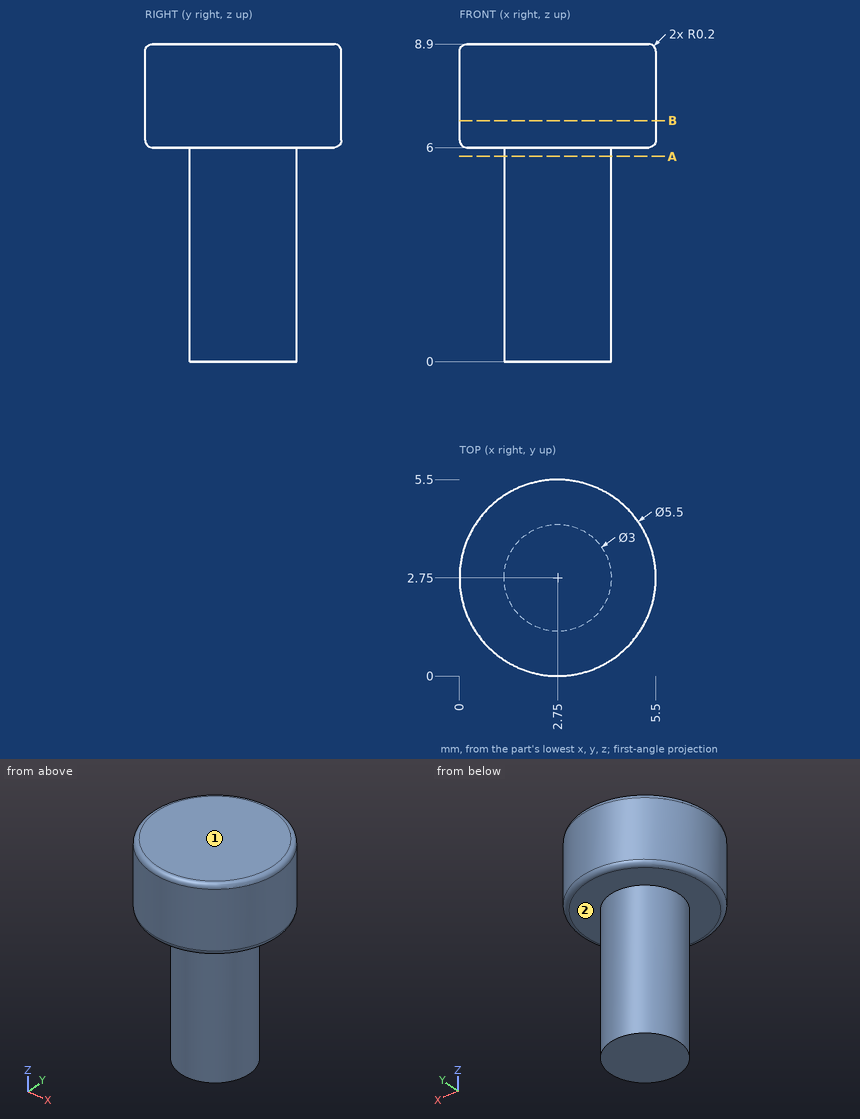
Could you check a few things on this drawing? It's one solid part, dimensions in mm from its lowest x, y, z. A direction names the side the tool comes from. Give positions to 0.01 mm unless a question says otherwise; leave off trailing zeros. Write each loop counter-clockwise with the first axis right and the second up, starting at its lowest first coordinate (ties: lowest second). Pieces come first, ordered by that corner, then holes. Notation, with made-up numbers: (85.5, -20.5) -> (133.5, -20.5) arc R8 cw to (133.5, -14.5) -> close; hole circle Ø9 at (40.25, 55.25). An arc over 180 degrees is marked (long way). Answer as CSV lines item,"result". Start each with the question number.
(1) If we section it at A-A, the plane z = 5.75: Write out the boundary of the cut face in (x, y).
(2) Which directions (+Z, -Z, +X, -X, +Y, -Y) give clear straight access to the entire face, cutting with the end or side of a thin tool? Please do the marked faces 1 and 2.
(3) I'm going to push flat-ended pins straight in: pin 1 Ø1 at (y, z) = (2.5, 1.5) entering from -X; pin 2 Ø3 at (y, z) = (1.5, 5) entering from +X; pin 3 Ø1 at (x, z) = (4, 1.5) entering from +Y. Where does each tip first touch, or does it pass through?
(4) Please list where these lines run through material, in increasing order: line 1 (Z direction, x = 2.5, y = 4.9); line 2 (X direction, y = 3.3, z = 0.75); line 3 (Y direction, x = 3.1, z = 3).
(5) If we section it at B-B, the plane z = 6.75: Write out the boundary of the cut face in (x, y).
Answer list:
1,outline,"circle Ø3 at (2.75, 2.75)"
2,face 1,"+Z, +X, -X, +Y, -Y"
2,face 2,"-Z"
3,pin 1,"x = 1.25"
3,pin 2,"x = 5.48"
3,pin 3,"y = 4.05"
4,line 1,"6 to 8.9"
4,line 2,"1.35 to 4.15"
4,line 3,"1.29 to 4.21"
5,outline,"circle Ø5.5 at (2.75, 2.75)"
